Autodesk Inventor part; units mm, degrees
ref_plane "YZ Plane" through (0, 0, 0) normal (1, 0, 0) x (0, 1, 0)
ref_plane "XZ Plane" through (0, 0, 0) normal (0, 1, 0) x (-1, 0, 0)
ref_plane "XY Plane" through (0, 0, 0) normal (0, 0, 1) x (1, 0, 0)
sketch "Sketch1" plane through (0, 0, 0) normal (0, 1, 0) x (-1, 0, 0)
  line L0 (-12.6881, -33.1691) -> (13.3119, -33.1691)
  line L1 (13.3119, -33.1691) -> (13.3119, 11.8309)
  line L2 (13.3119, 11.8309) -> (-12.6881, 11.8309)
  line L3 (-12.6881, 11.8309) -> (-12.6881, -33.1691)
  point P0 (0, 0)
  dimension "d0" = 45
  dimension "d1" = 26
extrude "Extrusion1" add sketch "Sketch1" along normal blind 4
sketch "Sketch2" plane through (0, 0, 0) normal (0, -1, 0) x (1, 0, 0)
  line L0 (-13.3119, 11.8309) -> (12.6881, 11.8309)
  line L1 (12.6881, 11.8309) -> (8.6881, 11.8309)
  line L2 (8.6881, 11.8309) -> (8.6881, -13.1691)
  line L3 (8.6881, -13.1691) -> (12.6881, -13.1691)
  line L4 (12.6881, -13.1691) -> (12.6881, 11.8309)
  point P0 (0, 0)
  point P1 (10.6881, -13.1691)
  dimension "d4" = 4
  dimension "d5" = 25
extrude "Extrusion2" add sketch "Sketch2" along normal blind 30
sketch "Sketch4" plane through (8.6881, 0, -13.1691) normal (-1, 0, 0) x (0, 0, 1)
  circle A0 centre (12, -17) radius 5
  line L0 (25, -30) -> (0, -30)
  line L1 (25, 0) -> (25, -30)
  point P0 (13.1691, 0)
  dimension "d8" = 10
  dimension "d9" = 13
  dimension "d10" = 13
extrude "Extrusion3" cut sketch "Sketch4" against normal through all
sketch "Sketch5" plane through (8.6881, 0, -13.1691) normal (-1, 0, 0) x (0, 0, 1)
  circle A0 centre (12, -9) radius 1.5
  circle A1 centre (12, -25) radius 1.5
  circle A2 centre (20, -17) radius 1.5
  circle A3 centre (4, -17) radius 1.5
  circle A4 centre (12, -17) radius 5
  point P0 (13.1691, 0)
  dimension "d13" = 3
  dimension "d14" = 3
  dimension "d15" = 3
  dimension "d16" = 3
  dimension "d17" = 8
  dimension "d19" = 8
  dimension "d20" = 8
  dimension "d21" = 8
  dimension "d22" = 8
  dimension "d23" = 8
  dimension "d24" = 8
extrude "Extrusion4" cut sketch "Sketch5" against normal through all contours A0 | A1 | A2 | A3
sketch "Sketch9" plane through (-13.3119, 4, 11.8309) normal (0, 0, 1) x (1, 0, 0)
  line L0 (0, -4) -> (0, 0)
  line L1 (26, -4) -> (26, -34)
  line L2 (0, 0) -> (26, 0)
  line L3 (26, 0) -> (26, -34)
  line L4 (26, -34) -> (0, -34)
  line L5 (0, -34) -> (0, 0)
  point P0 (13.3119, -4)
extrude "Extrusion6" add sketch "Sketch9" along normal blind 4
fillet "Fillet3" radius 5 3 edges at (-13.3119, -30, 13.8309) (10.6881, -30, -13.1691) (-2.3119, 0, 11.8309)
fillet "Fillet4" radius 8 1 edges at (-0.3119, 4, 15.8309)
fillet "Fillet5" radius 1.5 3 edges at (8.6881, -1.4645, 10.3664) (8.6881, 0, -3.1691) (8.6881, -17.5, 11.8309)
sketch "Sketch10" plane through (12.6881, 0, -33.1691) normal (0, 0, -1) x (-1, 0, 0)
  line L0 (0, 4) -> (26, 4)
  line L1 (0, 4) -> (26, 4)
  line L2 (26, 4) -> (26, -26)
  line L3 (26, -26) -> (0, -26)
  line L4 (0, -26) -> (0, 4)
  point P0 (12.6881, 0)
  dimension "d44" = 30
extrude "Extrusion7" add sketch "Sketch10" along normal blind 5
sketch "Sketch12" plane through (12.6881, 0, -38.1691) normal (0, 0, -1) x (-1, 0, 0)
  circle A0 centre (5, -3) radius 1.3
  circle A1 centre (21, -3) radius 1.3
  circle A2 centre (5, -21) radius 1.3
  circle A3 centre (21, -21) radius 1.3
  circle A4 centre (21, -12) radius 1.3
  line L0 (26, -26) -> (26, 4)
  line L1 (0, 4) -> (0, -26)
  line L2 (26, 4) -> (0, 4)
  line L3 (0, -26) -> (26, -26)
  circle A5 centre (5, -12) radius 1.3
  circle A6 centre (13, -21) radius 1.3
  circle A7 centre (13, -12) radius 1.3
  circle A8 centre (13, -3) radius 1.3
  point P0 (12.6881, 0)
  dimension "d47" = 2.6
  dimension "d48" = 2.6
  dimension "d49" = 2.6
  dimension "d50" = 2.6
  dimension "d51" = 2.6
  dimension "d52" = 5
  dimension "d53" = 5
  dimension "d54" = 5
  dimension "d55" = 5
  dimension "d56" = 7
  dimension "d57" = 7
  dimension "d58" = 16
  dimension "d59" = 5
  dimension "d60" = 5
  dimension "d61" = 5
  dimension "d64" = 2.6
  dimension "d65" = 16
  dimension "d66" = 5
  dimension "d81" = 2.6
  dimension "d82" = 2.6
  dimension "d83" = 2.6
  dimension "d84" = 5
  dimension "d85" = 13
  dimension "d86" = 13
  dimension "d87" = 13
  dimension "d88" = 7
  dimension "d89" = 16
extrude "Extrusion8" cut sketch "Sketch12" against normal up to surface (5 mm away) contours A0 | A1 | A2 | A3 | A4 | A5 | A6 | A7 | A8
sketch "Sketch13" plane through (0, 4, 0) normal (0, 1, 0) x (1, 0, 0)
  circle A0 centre (4.6881, 30.1691) radius 1.5
  circle A1 centre (4.6881, 15.1691) radius 1.5
  circle A2 centre (-5.3119, 30.1691) radius 1.5
  circle A3 centre (-5.3119, 15.1691) radius 1.5
  line L0 (-13.3119, 38.1691) -> (12.6881, 38.1691)
  line L1 (12.6881, 38.1691) -> (12.6881, -7.8309)
  point P0 (0, 0)
  dimension "d67" = 3
  dimension "d68" = 3
  dimension "d69" = 3
  dimension "d70" = 3
  dimension "d71" = 10
  dimension "d72" = 15
  dimension "d73" = 15
  dimension "d74" = 8
  dimension "d75" = 8
  dimension "d76" = 8
  dimension "d77" = 8
  dimension "d78" = 10
extrude "Extrusion9" cut sketch "Sketch13" against normal through all
chamfer "Chamfer3" distance 2 angle 45 4 edges at (3.1881, 4, -30.1691) (-6.8119, 4, -30.1691) (3.1881, 4, -15.1691) (-6.8119, 4, -15.1691)
sketch "Sketch14" plane through (-13.3119, 4, 15.8309) normal (0, 0, 1) x (1, 0, 0)
  circle A0 centre (6, -16) radius 1.3
  circle A1 centre (18, -16) radius 1.3
  circle A2 centre (6, -26) radius 1.3
  circle A3 centre (18, -26) radius 1.3
  line L0 (26, -34) -> (26, -8)
  line L1 (0, -8) -> (0, -29)
  line L2 (5, -34) -> (26, -34)
  point P0 (13.3119, -4)
  dimension "d93" = 2.6
  dimension "d94" = 2.6
  dimension "d95" = 2.6
  dimension "d96" = 2.6
  dimension "d97" = 8
  dimension "d98" = 8
  dimension "d99" = 6
  dimension "d100" = 6
  dimension "d101" = 8
  dimension "d102" = 8
  dimension "d103" = 10
  dimension "d104" = 10
extrude "Extrusion10" cut sketch "Sketch14" against normal up to surface (4 mm away)
sketch "Sketch15" plane through (0, 4, 0) normal (0, 1, 0) x (1, 0, 0)
  circle A0 centre (-6.3119, 9.1691) radius 1.3
  circle A1 centre (-6.3119, -3.8309) radius 1.3
  circle A2 centre (4.6881, -3.8309) radius 1.3
  circle A3 centre (4.6881, 9.1691) radius 1.3
  line L0 (12.6881, 38.1691) -> (12.6881, -7.8309)
  line L1 (-13.3119, -7.8309) -> (-13.3119, 38.1691)
  line L2 (-13.3119, 38.1691) -> (12.6881, 38.1691)
  point P0 (0, 0)
  dimension "d107" = 2.6
  dimension "d108" = 2.6
  dimension "d109" = 2.6
  dimension "d110" = 2.6
  dimension "d111" = 8
  dimension "d112" = 8
  dimension "d113" = 7
  dimension "d114" = 7
  dimension "d115" = 13
  dimension "d116" = 13
  dimension "d117" = 29
  dimension "d118" = 29
extrude "Extrusion11" cut sketch "Sketch15" against normal up to surface (4 mm away)
sketch "Sketch18" plane through (12.6881, -25, -13.1691) normal (1, 0, 0) x (0, 0, -1)
  line L0 (-20, 25) -> (0, 25)
  line L1 (0, 25) -> (-2, 25)
  line L2 (-2, 25) -> (-2, 16.5)
  line L3 (-2, 16.5) -> (0, 16.5)
  line L4 (0, 16.5) -> (0, 25)
  point P0 (-13.1691, 25)
  point P1 (-2, 25)
  dimension "d124" = 8.5
  dimension "d125" = 2
extrude "Extrusion13" cut sketch "Sketch18" against normal through all
chamfer "Chamfer4" distance 2 angle 45 1 edges at (10.6881, -8.5, -13.1691)
sketch "Sketch19" plane through (0, 4, 0) normal (0, 1, 0) x (1, 0, 0)
  circle A0 centre (-0.3119, 22.6691) radius 1.3
  line L0 (-13.3119, 38.1691) -> (12.6881, 38.1691)
  line L1 (12.6881, 38.1691) -> (12.6881, -7.8309)
  point P0 (0, 0)
  dimension "d131" = 2.6
  dimension "d132" = 15.5
  dimension "d133" = 13
extrude "Extrusion14" cut sketch "Sketch19" against normal through all
equation "\"d78\" = d71"
properties part number "probe_block_R" material "ABS Plastic"
Work out the finished part from the listing and answer in its coordinate system (mm). A direction names the side the tool comes from. Give positions to 0.01 mm unless a question says otherwise; leave off trailing zeros. Loops run counter-clockwise (first coordinate to the right, second up) from the corner with the lowest first, then second, coordinate; pieces in that order, holes last. Notation, with made-up numbers: (-24, 43) -> (16, 43) arc R24 ccw to (16, 82) -> close; hole circle Ø4 at (-23.75, 15). An arc over 180 degrees is marked (long way). Use a Markdown table: item, result. Add a question column.
1. Flat-ended cylindrical pins translate along their axes: pin 1 Ø1.6 at (x, y) = (-7.31, -12) entering from +Z; pin 2 Ø1.5 at (x, z) = (-10, -23) entering from -Y; pin 3 Ø12 at (y, z) = (-9, -1) entering from -X. Find the tip coordinate at first contact, or state that the pin passes through.
2. Section A-A on y = -17 is taken. Determine the outline of the cut face in (x, z), and give its area (3 significant figures).
3. Section C-C on z = -5.5 is taken. Determine the outline of the cut face in (x, y).
4. Section D-D on x = -10.75 is taken. Determine the outline of the cut face in (y, z), and give its area (3 significant figures).
5. Determine the mould class of faces 1 (the cylindrical face through (7.86, -10.71, -35.7)), 2 (the flat face through (0, 0, -13)) for opening direction X: released by +X, released by -X, zero draft, split by the parting line, or undercut.
6. For faces 3 (the flat face through (10.66, -9.51, -12.18)), 4 (the flat face through (0, -26, -36)), 5 (the cylindrical face through (-0.14, -1.71, -35.7)), 6 (the cylindrical face through (-2.9, -1.4, 10.3)), determine the directions among +Z, -Z, +X, -X, +Y, -Y from which every point of the face is accessible in a straight line to the end or side of a thin tool.
7. Find the intervals of material crossed by probe 1 along Z at (x, y) = (11.25, -19.5); probe 2 along Z at (x, y) = (2, -20); probe 3 along Z at (x, y) = (9, -6.5), in increasing order.
8. Section B-B on x = -1 is taken. Determine the outline of the cut face in (y, z).
Results below:
| question | item | result |
|---|---|---|
| 1 | pin 1 | stops at z = -33.17 |
| 1 | pin 2 | stops at y = 0 |
| 1 | pin 3 | stops at x = 8.69 |
| 2 | outline | (-13.31, -38.17) -> (12.69, -38.17) -> (12.69, -33.17) -> (-13.31, -33.17) -> close; (-13.31, 11.83) -> (7.19, 11.83) arc R1.5 cw to (8.69, 10.33) -> (8.69, 8.33) -> (12.69, 8.33) -> (12.69, 15.83) -> (-13.31, 15.83) -> close; (8.69, -13.17) -> (12.69, -13.17) -> (12.69, -10.67) -> (8.69, -10.67) -> close; (8.69, -7.67) -> (12.69, -7.67) -> (12.69, -6.17) -> (8.69, -6.17) -> close; (8.69, 3.83) -> (12.69, 3.83) -> (12.69, 5.33) -> (8.69, 5.33) -> close |
| 2 | area | 270 mm^2 |
| 3 | outline | (-13.31, 0) -> (7.19, 0) arc R1.5 cw to (8.69, -1.5) -> (8.69, -14.5) -> (12.69, -14.5) -> (12.69, 4) -> (-13.31, 4) -> close; (8.69, -30) -> (12.69, -30) -> (12.69, -19.5) -> (8.69, -19.5) -> close |
| 4 | outline | (-29.37, 11.83) -> (-5, 11.83) arc R5 cw to (0, 6.83) -> (0, -33.17) -> (-26, -33.17) -> (-26, -38.17) -> (4, -38.17) -> (4, 7.83) arc R8 ccw to (-4, 15.83) -> (-29.37, 15.83) -> close |
| 4 | area | 455 mm^2 |
| 5 | face 1 | undercut |
| 5 | face 2 | zero draft |
| 6 | face 3 | +X, -X |
| 6 | face 4 | -Z, +X, -X, -Y |
| 6 | face 5 | -Z |
| 6 | face 6 | -X, -Y |
| 7 | probe 1 | z = -38.17 to -33.17, -13.17 to -5.5, 3.16 to 15.83 |
| 7 | probe 2 | z = -38.17 to -33.17, 11.83 to 15.83 |
| 7 | probe 3 | z = -38.17 to -33.17, -11.17 to 15.83 |
| 8 | outline | (-30, 11.83) -> (-5, 11.83) arc R5 cw to (0, 6.83) -> (0, -21.57) -> (4, -21.57) -> (4, 7.83) arc R8 ccw to (-4, 15.83) -> (-30, 15.83) -> close; (-26, -38.17) -> (-22.1, -38.17) -> (-22.1, -33.17) -> (-26, -33.17) -> close; (-19.9, -38.17) -> (-13.1, -38.17) -> (-13.1, -33.17) -> (-19.9, -33.17) -> close; (-10.9, -38.17) -> (-4.1, -38.17) -> (-4.1, -33.17) -> (-10.9, -33.17) -> close; (-1.9, -38.17) -> (4, -38.17) -> (4, -23.77) -> (0, -23.77) -> (0, -33.17) -> (-1.9, -33.17) -> close |
